from build123d import *

# Parameters (mm, degrees)
SKETCH1_R           = 2
BOSS_EXTRUDE1_DEPTH = 24.13
SKETCH2_R           = 11.43
CUT_EXTRUDE1_DEPTH  = 57.932251879


with BuildPart() as part:
    # Sketch1 → Boss-Extrude1 (new body)
    with BuildSketch(Plane(origin=(0, 0, 0), x_dir=(1, 0, 0), z_dir=(0, 1, 0))):
        with BuildLine():
            Line((7.99846, 0), (41.02154, 0))
            ThreePointArc((41.02154, 0), (46.677305305, 2.342694695), (49.02, 7.99846))
            Line((49.02, 7.99846), (49.02, 8.00354))
            ThreePointArc((49.02, 8.00354), (46.677305305, 13.659305305), (41.02154, 16.002))
            Line((41.02154, 16.002), (7.99846, 16.002))
            ThreePointArc((7.99846, 16.002), (2.342694695, 13.659305305), (0, 8.00354))
            Line((0, 8.00354), (0, 7.99846))
            ThreePointArc((0, 7.99846), (2.342694695, 2.342694695), (7.99846, 0))
        make_face()
        with Locations(Location((4, 8.001, 0), (0, 0, 90))):
            Circle(SKETCH1_R, mode=Mode.SUBTRACT)
        with Locations(Location((45.02, 8.001, 0), (0, 0, 90))):
            Circle(SKETCH1_R, mode=Mode.SUBTRACT)
    extrude(amount=BOSS_EXTRUDE1_DEPTH)

    # Sketch2 → Cut-Extrude1 (cut, through all)
    with BuildSketch(Plane.XY):
        with Locations((24.51, 24.13)):
            Circle(SKETCH2_R)
    extrude(amount=-CUT_EXTRUDE1_DEPTH, mode=Mode.SUBTRACT)


solid = part.part
Can you work these out from the model? Positions are in its coordinate system, mm. Coordinates: 2 decimals unless noted, no trailing zeros. Order: outer loops, then holes, each group sorted by start corner. A loop starts at its lowest first (then second) coordinate and runs counter-clockwise, first axis right, second up. Notation, with made-up numbers: (15, 35.25) - (66, 35.25) arc R14 cw to (66, 54.25) - close; hole circle Ø11 at (43.5, -25). An arc over 180 degrees is marked (long way). Answer as a JSON object with one key per item and string values. Group by question number.
Q1. We'd pull the mould along X, two halves only. Please class faces 1 (the face through (2.281, 11.896, -2.405)), 2 (the face through (24, 9, 0)), 3 (the face through (5.2, 11.9, -6.4)): +X half, -X half, draft (parallel to the pull), parting line (faces both ways), or undercut.
Q2. Imagine slicing it at A-A (y = 17.75). Give the number of separate pieces and of enclosed holes in the cut face, and give its area (3 significant figures).
Q3. Imagine slicing it at B-B (x = 4). Please give me the cut outline in (y, z), and give its area (3 significant figures).
Q4. I need wall thicknesses on line 1 (X direction, y = 20, z = -9.75); line 2 (X direction, y = 19.25, z = -9.5); line 3 (X direction, y = 19.75, z = -11.5). Which ranges of each line are inside material? Lowest first, please. Write a range as from..to.
Q5. Will this pin go through, and if not, where does the flat tip stop? P1, Ø5, axis at y = 5, z = -12, coming from the +X side.
Q6. Imagine slicing it at D-D (z = -8.5). Please give me the cut outline in (x, y).
Determined:
{
 "1": {"face 1": "-X half", "face 2": "draft", "face 3": "undercut"},
 "2": {"separate pieces": "2", "enclosed holes": "2", "area": "401 mm2"},
 "3": {"outline": "(0, -14.93) - (24.13, -14.93) - (24.13, -10) - (0, -10) - close; (0, -6) - (24.13, -6) - (24.13, -1.07) - (0, -1.07) - close", "area": "238 mm2"},
 "4": {"line 1": "x = 0.19..3.03, 4.97..13.85, 35.17..44.05, 45.99..48.83", "line 2": "x = 0.14..2.68, 5.32..14.17, 34.85..43.7, 46.34..48.88", "line 3": "x = 0.8..13.95, 35.07..48.22"},
 "5": {"P1": "stops at x = 48.88"},
 "6": {"outline": "(0.02, 0) - (2.06, 0) - (2.06, 24.13) - (0.02, 24.13) - close; (5.94, 0) - (43.08, 0) - (43.08, 24.13) - (35.94, 24.13) arc R11.43 cw to (13.08, 24.13) - (5.94, 24.13) - close; (46.96, 0) - (49, 0) - (49, 24.13) - (46.96, 24.13) - close"}
}
